Work out the finished part from the listing and answer in its coordinate system (mm). Round coordinates to 2 decimals unless told otherwise and drop trailing zeros. Write each loop counter-clockwise with the first axis right and the second up, starting at its lowest first coordinate (ties: lowest second). Pieces come first, ordered by that corner, then holes. Notation, with made-up numbers: M -15.75,25 L 0.25,25 A17 ccw 0.25,33 Z; hole C 78,-20.5 d11. An arc over 180 degrees is marked long. One line per item, written item: value. Start each with the question number.
Q1. Find section C-C (z = 536). Write down the section's boundary in (x, y).
Q2. Consider probe 1 along X at (y, z) = (-6, 365); probe 2 along Z at (x, y) = (5, 1). Determine where each line is inside the solid, lowest interval first.
Q3. Find section B-B (z = 385.5). Write down the section's boundary in (x, y), and give its area (3 significant figures).
Q4. Find section A-A (y = 0.5). Write down the section's boundary in (x, z).
Q5. Given pin 1 Ø12 at (y, z) = (-2, 518.5) entering from +X; pin 2 Ø1 at (x, z) = (5, 161) entering from +Y, each flat-ended and moving along its own axis, determine where each tip first touches the part or whether it passes through.
from build123d import *

# Parameters (mm, degrees)
F0_W     = 32.766
F0_H     = 32.766
F1_DEPTH = 660.4
F2_W     = 13.97
F2_H     = 13.97
F3_DEPTH = 647.7
F5_DEPTH = 66.294
F6_W     = 11.1841903999
F6_H     = 90.8770263195
F7_DEPTH = 96.266


with BuildPart() as f1:
    # F0 (on Top) → F1 (new body)
    with BuildSketch(Plane.XY):
        Rectangle(F0_W, F0_H)
    extrude(amount=F1_DEPTH)

    # F2 (on face) → F3 (cut)
    with BuildSketch(Plane.XY.offset(660.4)):
        with Locations((-6.985, 6.985)):
            Rectangle(F2_W, F2_H)
        with Locations((6.985, 6.985)):
            Rectangle(F2_W, F2_H)
        with Locations((6.985, -6.985)):
            Rectangle(F2_W, F2_H)
        with Locations((-6.985, -6.985)):
            Rectangle(F2_W, F2_H)
    extrude(amount=-F3_DEPTH, mode=Mode.SUBTRACT)

    # F4 (on face) → F5 (cut)
    with BuildSketch(Plane.XZ.offset(16.383)):
        with BuildLine():
            Line((0, 25.4), (0, 635))
            ThreePointArc((0, 635), (-4.4901280605, 636.8598719395), (-6.35, 641.35))
            Line((-6.35, 641.35), (-6.35, 19.05))
            ThreePointArc((-6.35, 19.05), (-4.4901280605, 23.5401280605), (0, 25.4))
        make_face()
        with BuildLine():
            Line((0, 635), (0, 647.7))
            ThreePointArc((0, 647.7), (-4.4901280605, 645.8401280605), (-6.35, 641.35))
            ThreePointArc((-6.35, 641.35), (-4.4901280605, 636.8598719395), (0, 635))
        make_face()
        with BuildLine():
            ThreePointArc((6.35, 641.35), (4.4901280605, 645.8401280605), (0, 647.7))
            Line((0, 647.7), (0, 635))
            ThreePointArc((0, 635), (4.4901280605, 636.8598719395), (6.35, 641.35))
        make_face()
        with BuildLine():
            ThreePointArc((6.35, 641.35), (4.4901280605, 636.8598719395), (0, 635))
            Line((0, 635), (0, 25.4))
            ThreePointArc((0, 25.4), (4.4901280605, 23.5401280605), (6.35, 19.05))
            Line((6.35, 19.05), (6.35, 641.35))
        make_face()
        with BuildLine():
            Line((0, 12.7), (0, 25.4))
            ThreePointArc((0, 25.4), (-4.4901280605, 23.5401280605), (-6.35, 19.05))
            ThreePointArc((-6.35, 19.05), (-4.4901280605, 14.5598719395), (0, 12.7))
        make_face()
        with BuildLine():
            ThreePointArc((6.35, 19.05), (4.4901280605, 23.5401280605), (0, 25.4))
            Line((0, 25.4), (0, 12.7))
            ThreePointArc((0, 12.7), (4.4901280605, 14.5598719395), (6.35, 19.05))
        make_face()
    extrude(amount=-F5_DEPTH, mode=Mode.SUBTRACT)

    # F6 (on face) → F7 (cut)
    with BuildSketch(Plane.YZ.offset(16.383)):
        with Locations((0, 517.8375393152)):
            Rectangle(F6_W, F6_H)
    extrude(amount=-F7_DEPTH, mode=Mode.SUBTRACT)


solid = f1.part
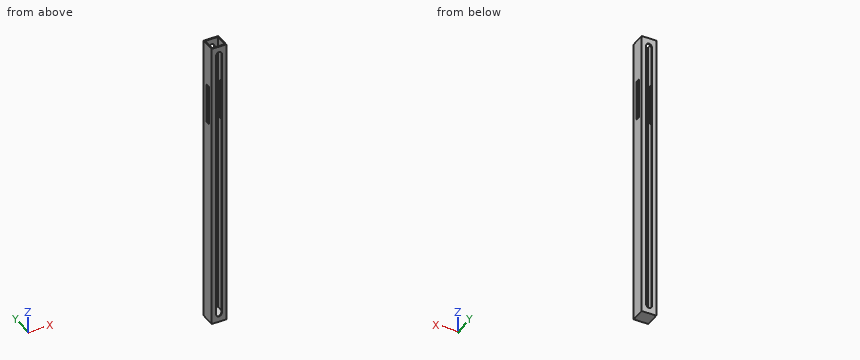
The answers:
1. outline: M -16.38,-16.38 L -6.35,-16.38 L -6.35,-13.97 L -13.97,-13.97 L -13.97,-5.59 L -16.38,-5.59 Z; M -16.38,5.59 L -13.97,5.59 L -13.97,13.97 L -6.35,13.97 L -6.35,16.38 L -16.38,16.38 Z; M 6.35,-16.38 L 16.38,-16.38 L 16.38,-5.59 L 13.97,-5.59 L 13.97,-13.97 L 6.35,-13.97 Z; M 6.35,13.97 L 13.97,13.97 L 13.97,5.59 L 16.38,5.59 L 16.38,16.38 L 6.35,16.38 Z
2. probe 1: -16.38 to -13.97, 13.97 to 16.38
2. probe 2: 0 to 12.7
3. outline: M -16.38,-16.38 L -6.35,-16.38 L -6.35,-13.97 L -13.97,-13.97 L -13.97,13.97 L -6.35,13.97 L -6.35,16.38 L -16.38,16.38 Z; M 6.35,-16.38 L 16.38,-16.38 L 16.38,16.38 L 6.35,16.38 L 6.35,13.97 L 13.97,13.97 L 13.97,-13.97 L 6.35,-13.97 Z
3. area: 232 mm2
4. outline: M -16.38,0 L 16.38,0 L 16.38,472.4 L 13.97,472.4 L 13.97,12.7 L -13.97,12.7 L -13.97,472.4 L -16.38,472.4 Z; M -16.38,563.28 L -13.97,563.28 L -13.97,660.4 L -16.38,660.4 Z; M 13.97,563.28 L 16.38,563.28 L 16.38,660.4 L 13.97,660.4 Z
5. pin 1: x = 16.38
5. pin 2: through
